from build123d import *

# Parameters (mm, degrees)
BOSS_EXTRUDE4_DEPTH          = 40
SKETCH18_R                   = 12.5
BOSS_EXTRUDE2_DEPTH          = 5
SKETCH19_R                   = 9.95
BOSS_EXTRUDE3_DEPTH          = 30
FILLET1_R                    = 10
M5_START                     = -139.716402581
M5_CLEARANCE_HOLE2_OUTLINE_R = 2.75
M5_CLEARANCE_HOLE2_DEPTH     = 7.727879289
CHAMFER1_SIZE                = 1


# Read off the part's stored shape, not the designer's step: M5 Clearance Hole2
with BuildPart() as part:
    # Sketch20 → Boss-Extrude4 (new body)
    with BuildSketch(Plane(origin=(0, 0, 0), x_dir=(1, 0, 0), z_dir=(0, 1, 0))):
        with BuildLine():
            Line((112.573466187, -234.162128136), (116.826154662, -227.98437444))
            ThreePointArc((116.826154662, -227.98437444), (133.75, -238.671414456), (151.467170814, -247.98437444))
            Line((151.467170814, -247.98437444), (154.690918215, -241.212561338))
            ThreePointArc((154.690918215, -241.212561338), (58.362499128, -159.166512646), (15.817691059, -40))
            Line((15.817691059, -40), (15, -40))
            Line((15, -40), (15, -20))
            Line((15, -20), (15, 0))
            Line((15, 0), (0, 0))
            Line((0, 0), (0, -20))
            Line((0, -20), (0, -40))
            Line((0, -40), (0.770372064, -40))
            ThreePointArc((0.770372064, -40), (34.68457338, -149.741891952), (112.573466187, -234.162128136))
        make_face()
    extrude(amount=BOSS_EXTRUDE4_DEPTH)

    # Sketch18 → Boss-Extrude2 (add)
    with BuildSketch(Plane.ZY):
        with Locations((20, 20)):
            Circle(SKETCH18_R)
    extrude(amount=BOSS_EXTRUDE2_DEPTH)

    # Sketch19 → Boss-Extrude3 (add)
    with BuildSketch(Plane.ZY.offset(5)):
        with Locations((20, 20)):
            Circle(SKETCH19_R)
    extrude(amount=BOSS_EXTRUDE3_DEPTH)

    # Fillet1
    fillet1_edges = [part.edges().sort_by_distance(p)[0] for p in [
        (7.5, 0, 0),
        (7.5, 40, 0),
    ]]
    fillet(fillet1_edges, radius=FILLET1_R)

    # M5 Clearance Hole2 outline → M5 Clearance Hole2 (cut)
    with BuildSketch(Plane(origin=(0, 0, 0), x_dir=(0.8660254037844398, 0, 0.499999999999998), z_dir=(0.49999999999999795, 0, -0.8660254037844399)).offset(M5_START)):
        with Locations((245.166604984, -30)):
            Circle(M5_CLEARANCE_HOLE2_OUTLINE_R)
        with Locations((225.166604984, -10)):
            Circle(M5_CLEARANCE_HOLE2_OUTLINE_R)
        with Locations((225.166604984, -30)):
            Circle(M5_CLEARANCE_HOLE2_OUTLINE_R)
        with Locations((245.166604984, -10)):
            Circle(M5_CLEARANCE_HOLE2_OUTLINE_R)
    extrude(amount=M5_CLEARANCE_HOLE2_DEPTH, mode=Mode.SUBTRACT)

    # Chamfer1
    chamfer1_edges = [part.edges().sort_by_distance(p)[0] for p in [
        (-35, 20, 10.05),
    ]]
    chamfer(chamfer1_edges, length=CHAMFER1_SIZE)


solid = part.part
Can you work these out from the model? Positions are in its coordinate system, mm. A direction names the side the tool comes from. Give positions to 0.01 mm unless a question says otherwise; leave off trailing zeros. Write each loop counter-clockwise with the first axis right and the second up, starting at its lowest first coordinate (ties: lowest second). Pieces come first, ordered by that corner, then holes. Notation, with made-up numbers: M 77,55.25 L 103,55.25 A13 cw 103,63.25 Z; hole C -36.75,-40 d9. An arc over 180 degrees is marked long. Answer in a Markdown table with one row per item. Add a question column.
Item 1: For pin 1 Ø1.5 at (y, z) = (34.5, 193) entering from -X; pin 2 Ø1 at (x, y) = (43.5, 31.5) entering from +Z; pin 3 Ø5 at (y, z) = (33.5, 111) entering from -X, each with a flat end and sliding along its axis, tell me the tip position at first contact or that it passes through.
Item 2: On a 3-axis mill with a long thin cutter (end or side, diameter ignored), from which of +Z, -Z, +X, -X, +Y, -Y can I reach the whole of each face in a straight line? I mean faces 1 (the flat face through (15, 20, 20)), 2 (the cylindrical face through (133.507, 19.72, 238.531)), 3 (the flat face through (-5, 9.9, 19)), 4 (the flat face through (153.056, 19.72, 244.646)), 5 (the flat face through (43, 40, 137)). Say none if no direction works.
Item 3: Imagine slicing it at A-A, the plane z = 20. Write out the boundary of the cut face in (x, y), plus the area to 3 significant figures.
Item 4: We'd pull the mould along Y, two halves only. Please class faces 6 (the cylindrical face through (126.737, 27.273, 230.103)), 7 (the cylindrical face through (-19.3, 13.95, 12.1)), 8 (the cylindrical face through (7.4, 37.15, 3.01)): released by +Y, released by -Y, zero draft, split by the parting line, or undercut.
Item 5: Imagine slicing it at D-D, the plane z = 79.5. Write out the boundary of the cut face in (x, y), plus the area to 3 significant figures.
Item 6: Please list where these lines run through material, in increasing order: L1, parallel to X at y = 3.5, z = 37; L2, parallel to X at y = 24, z = 179.5; L3, parallel to Z at x = 56, y = 13.5.
Item 7: Imagine slicing it at C-C, the plane x = 92.5. Write out the boundary of the cut face in (y, z), plus the area to 3 significant figures.
Item 8: Imagine slicing it at B-B, the plane x = -9. Write out the boundary of the cut face in (y, z), plus the area to 3 significant figures.
Evaluation:
| question | item | result |
|---|---|---|
| 1 | pin 1 | stops at x = 65.24 |
| 1 | pin 2 | stops at z = 164.72 |
| 1 | pin 3 | stops at x = 15.53 |
| 2 | face 1 | -Z, +X, +Y, -Y |
| 2 | face 2 | +Z, +Y, -Y |
| 2 | face 3 | -X |
| 2 | face 4 | +Z, +X, +Y, -Y |
| 2 | face 5 | +Z, -Z, +X, -X, +Y |
| 3 | outline | M -35,11.05 L -34,10.05 L -5,10.05 L -5,7.5 L 0,7.5 L 0,0 L 15,0 L 15,40 L 0,40 L 0,32.5 L -5,32.5 L -5,29.95 L -34,29.95 L -35,28.95 Z |
| 3 | area | 1,320 mm² |
| 4 | face 6 | undercut |
| 4 | face 7 | split by the parting line |
| 4 | face 8 | released by +Y |
| 5 | outline | M 6.9,0 L 22.33,0 L 22.33,40 L 6.9,40 Z |
| 5 | area | 617 mm² |
| 6 | L1 | x = 0 to 15 |
| 6 | L2 | x = 54.67 to 74.03 |
| 6 | L3 | z = 155.68 to 181.2 |
| 7 | outline | M 0,198.8 L 40,198.8 L 40,218.86 L 0,218.86 Z |
| 7 | area | 802 mm² |
| 8 | outline | C 20,20 d19.9 |
| 8 | area | 311 mm² |
